Geometry: final body of the model. Coordinates: model frame, mm. A direction names the side the tool comes from. Give positions to 0.01 mm unless a question says otherwise; leave off trailing zeros. Write each loop counter-clockwise with the first axis right and the second up, starting at its lowest first coordinate (ties: lowest second). Pieces come first, ordered by that corner, then holes. Notation, with made-up numbers: (-38.5, 5.5) -> (-11.5, 5.5) arc R29 cw to (-11.5, 29.5) -> close; hole circle Ø3 at (30.25, 83.5). An arc over 180 degrees is marked (long way). Answer as a JSON object with one key per item and string values. Group by question number.
(1) Set-up query: faces 1 (the face through (-1.82, 0.86, -0.51)), 2 (the face through (-2.36, 1, -1)), 3 (the face through (0, 1, -1)). Return all of +Z, -Z, +X, -X, +Y, -Y with unobstructed straight access to the full face (end or side cutting, diameter ignored); none if empty.
(2) Draft query along Z for faces 4 (the face through (3.93, -0.27, -1.22)), 5 (the face through (8, 0, 0)), 6 (the face through (-1.82, -0.87, -0.49)). Return one class per face: +Z half, -Z half, draft (parallel to the pull), parting line (faces both ways), or undercut.
(3) Material intervals for probe 1 along Z at (x, y) = (1.75, -0.75); probe 2 along X at (y, z) = (-1.35, 0.2); probe 3 along Z at (x, y) = (-2, 0.1), sorted ascending.
(4) Section query B-B on x = 4. Output: boundary loops of the cut face in (y, z).
(5) Contact query for a flat-ended pin moving along its axis: pin 1 Ø2 at (x, z) = (7, 0.5) entering from +Y. Output: stop coordinate, or through.
(6) Section query A-A on x = -0.25. Output: boundary loops of the cut face in (y, z), plus the area to 3 significant figures.
Autodesk Inventor part; units mm, degrees
ref_plane "SCW_XY" through (0, 0, 0) normal (1, 0, 0) x (0, 0, -1)
ref_plane "SCW_YZ" through (0, 0, 0) normal (0, 0, -1) x (0, 1, 0)
ref_plane "SCW_ZX" through (0, 0, 0) normal (0, 1, 0) x (1, 0, 0)
sketch "Sketch_1" plane through (0, 0, 0) normal (0, 0, 1) x (1, 0, 0)
  line L0 (8, 0) -> (-2.36, 0)
  line L1 (-2.36, 0) -> (-2.36, 2)
  line L2 (-2.36, 2) -> (-2.11, 2.25)
  line L3 (-2.11, 2.25) -> (0, 2.25)
  line L4 (0, 2.25) -> (0, 1.25)
  line L5 (0, 1.25) -> (7.7565, 1.25)
  line L6 (7.7565, 1.25) -> (8, 1.0065)
  line L7 (8, 1.0065) -> (8, 0)
  line L8 (8, 0) -> (-2.36, 0)
revolve "Revolution1" add sketch "Sketch_1" angle 360 about axis through (8, 0, 0) along (1, 0, 0)
thread "Thread1"
sketch "Sketch_2" plane through (-2.36, 0, 0) normal (1, 0, 0) x (0, 0, -1)
  line L0 (-1, -0.5774) -> (0, -1.1547)
  line L1 (0, -1.1547) -> (1, -0.5774)
  line L2 (1, -0.5774) -> (1, 0.5774)
  line L3 (1, 0.5774) -> (0, 1.1547)
  line L4 (0, 1.1547) -> (-1, 0.5774)
  line L5 (-1, 0.5774) -> (-1, -0.5774)
extrude "Extrusion1" cut sketch "Sketch_2" along normal blind 1.1
sketch "Sketch_5" plane through (0, 0, 0) normal (0, 0, 1) x (1, 0, 0)
  line L0 (-0.6826, 0) -> (-1.26, 0)
  line L1 (-1.26, 0) -> (-1.26, 1)
  line L2 (-1.26, 1) -> (-0.6826, 0)
  line L3 (-0.6826, 0) -> (-1.26, 0)
revolve "Revolution2" cut sketch "Sketch_5" angle 360 about axis through (-0.6826, 0, 0) along (1, 0, 0)
ref_plane "SCW_XY" through (0, 0, 0) normal (1, 0, 0) x (0, 0, -1)
ref_plane "SCW_YZ" through (0, 0, 0) normal (0, 0, -1) x (0, 1, 0)
ref_plane "SCW_ZX" through (0, 0, 0) normal (0, 1, 0) x (1, 0, 0)
properties part number "M2.5" material "アルミニウム 6061"
Answer list:
{
 "1": {"face 1": "-X", "face 2": "+Z, -Z, -X, +Y, -Y", "face 3": "+X"},
 "2": {"face 4": "parting line", "face 5": "draft", "face 6": "undercut"},
 "3": {"probe 1": "-1 to 1", "probe 2": "-2.36 to 0", "probe 3": "-2.25 to -1, 1 to 2.25"},
 "4": {"outline": "circle Ø2.5 at (0, 0)"},
 "5": {"pin 1": "y = 1.25"},
 "6": {"outline": "circle Ø4.5 at (0, 0)", "area": "15.9 mm2"}
}
